Design review of the part built by this model. Coordinates are the model's own, in mm. A direction names the side the tool comes from. Coordinates: 2 decimals unless noted, no trailing zeros. Loops run counter-clockwise (first coordinate to the right, second up) from the corner with the lowest first, then second, coordinate; pieces in that order, holes last. Notation, with made-up numbers: (36.25, 47) -> (78.25, 47) arc R23 cw to (78.25, 86) -> close; hole circle Ø1 at (-33, 68.25). An arc over 180 degrees is marked (long way). Use one line per item in the form item = value. Start each with the question number.
1. Consider section C-C (z = 466). State the section outline as (x, y) points, then the cut area to 3 significant figures.
2. Wall thickness on line 1 (Z direction, x = 833, y = -387); line 2 (Y direction, x = 249.5, z = -290); line 3 (Z direction, x = 970, y = -8): over which ranges is each line inside the solid? List them lowest first. Write a range as from..to.
3. For pin 1 (12.5 mm diameter, centred on y = 204.5, z = 171, fed in from +X); pin 2 (6 mm diameter, centred on y = -640, z = -546, fed in from +X); pin 3 (3 mm diameter, centred on x = 165, z = -67.5, fed in from -Y), all flat-tipped, find the tip position at first contact; note any pin that passes through.
4. Machinability: for faces 1 (the face through (995, -792, -966.353)), 2 (the face through (923, -716, -1220.353)), 3 (the face through (467, -57, 153.79)), which of the approach directions +Z, -Z, +X, -X, +Y, -Y give a long, thin tool a straight path to every point of the face, cutting with its end or side? Answer none if there is none.
5. Consider section A-A (x = 362.5). State the section outline as (y, z) points, then the cut area to 3 significant figures.
6. Consider section D-D (z = -1044.5). State the section outline as (x, y) points, then the cut area to 3 significant figures.
7. Consider section B-B (y = 119). State the section outline as (x, z) points.
8. The part is to be moulded in two halves that separate along Y. For faces 4 (the face through (467, -57, -453.211)), 5 (the face through (100, -716, -1220.353)), 6 (the face through (501, -808.5, -27)), 7 (the face through (29.83, -780.18, -1091.57)), say which applies: released by +Y, released by -Y, zero draft, split by the parting line, or undercut.
from build123d import *

# Parameters (mm, degrees)
F0_W     = 1524
F0_H     = 1905
F1_DEPTH = 1016
F2_T     = -2.54
F3_W     = 1518.92
F3_H     = 25.4
F4_DEPTH = 942.34
F5_R     = 97.372943
F6_DEPTH = 254


with BuildPart() as f1:
    # F0 (on Right) → F1 (new body)
    with BuildSketch(Plane.YZ):
        with Locations((-46.499569, -13.852631)):
            Rectangle(F0_W, F0_H)
    extrude(amount=F1_DEPTH)

    # F2
    f2_openings = [f1.faces().sort_by_distance(p)[0] for p in [
        (1016, -46.499569, -13.852631),
    ]]
    offset(amount=F2_T, openings=f2_openings)

    # F3 (on face) → F4 (join)
    with BuildSketch(Plane.YZ.offset(2.54)):
        with Locations((-46.499569, -465.910843)):
            Rectangle(F3_W, F3_H)
        with Locations((-46.499569, 542.111227)):
            Rectangle(F3_W, F3_H)
        with Locations((-46.499569, 166.490295)):
            Rectangle(F3_W, F3_H)
        with Locations((-46.499569, -97.188047)):
            Rectangle(F3_W, F3_H)
    extrude(amount=F4_DEPTH)

    # F5 (on face) → F6 (join)
    with BuildSketch(Plane(origin=(0, 0, -966.352631), x_dir=(1, 0, 0), z_dir=(0, 0, -1))):
        with Locations((924.561083, 714.374423)):
            Circle(F5_R)
        with Locations((924.561083, -616.585577)):
            Circle(F5_R)
        with Locations((101.601083, 714.374423)):
            Circle(F5_R)
        with Locations((101.601083, -616.585577)):
            Circle(F5_R)
    extrude(amount=F6_DEPTH)


solid = f1.part
Geometry check:
q1.outline = (0, -808.5) -> (1016, -808.5) -> (1016, -805.96) -> (2.54, -805.96) -> (2.54, 712.96) -> (1016, 712.96) -> (1016, 715.5) -> (0, 715.5) -> close
q1.area = 9,020 mm²
q2.line_1 = -966.35..-963.81, -478.61..-453.21, -109.89..-84.49, 153.79..179.19, 529.41..554.81, 936.11..938.65
q2.line_2 = -808.5..-805.96, 712.96..715.5
q2.line_3 = -966.35..-963.81, 936.11..938.65
q3.pin_1 = 944.88
q3.pin_2 = 2.54
q3.pin_3 = -808.5
q4.face_1 = -Z, +X, -Y
q4.face_2 = -Z, +X, -X, +Y, -Y
q4.face_3 = +X
q5.outline = (-808.5, -966.35) -> (715.5, -966.35) -> (715.5, 938.65) -> (-808.5, 938.65) -> close; hole (-805.96, -963.81) -> (712.96, -963.81) -> (712.96, -478.61) -> (-805.96, -478.61) -> close; hole (-805.96, -453.21) -> (712.96, -453.21) -> (712.96, -109.89) -> (-805.96, -109.89) -> close; hole (-805.96, -84.49) -> (712.96, -84.49) -> (712.96, 153.79) -> (-805.96, 153.79) -> close; hole (-805.96, 179.19) -> (712.96, 179.19) -> (712.96, 529.41) -> (-805.96, 529.41) -> close; hole (-805.96, 554.81) -> (712.96, 554.81) -> (712.96, 936.11) -> (-805.96, 936.11) -> close
q5.area = 172,000 mm²
q6.outline = circle Ø194.75 at (101.6, -714.37); circle Ø194.75 at (101.6, 616.59); circle Ø194.75 at (924.56, -714.37); circle Ø194.75 at (924.56, 616.59)
q6.area = 119,000 mm²
q7.outline = (0, -966.35) -> (1016, -966.35) -> (1016, -963.81) -> (2.54, -963.81) -> (2.54, -478.61) -> (944.88, -478.61) -> (944.88, -453.21) -> (2.54, -453.21) -> (2.54, -109.89) -> (944.88, -109.89) -> (944.88, -84.49) -> (2.54, -84.49) -> (2.54, 153.79) -> (944.88, 153.79) -> (944.88, 179.19) -> (2.54, 179.19) -> (2.54, 529.41) -> (944.88, 529.41) -> (944.88, 554.81) -> (2.54, 554.81) -> (2.54, 936.11) -> (1016, 936.11) -> (1016, 938.65) -> (0, 938.65) -> close
q8.face_4 = undercut
q8.face_5 = zero draft
q8.face_6 = released by -Y
q8.face_7 = undercut
